```python
from build123d import *

# Parameters (mm, degrees)
SKETCH1_W           = 100
SKETCH1_H           = 100
SKETCH1_R           = 2.75
BOSS_EXTRUDE1_DEPTH = 4.3
SKETCH2_R           = 1.75
BOSS_EXTRUDE2_DEPTH = 4.3
FILLET1_R           = 10


with BuildPart() as part:
    # Sketch1 → Boss-Extrude1 (new body)
    with BuildSketch(Plane(origin=(0, 0, 0), x_dir=(1, 0, 0), z_dir=(0, 1, 0))):
        with Locations((50, 50)):
            Rectangle(SKETCH1_W, SKETCH1_H)
        with Locations((20, 80)):
            Circle(SKETCH1_R, mode=Mode.SUBTRACT)
        with Locations((80, 80)):
            Circle(SKETCH1_R, mode=Mode.SUBTRACT)
        with Locations((80, 20)):
            Circle(SKETCH1_R, mode=Mode.SUBTRACT)
        with Locations((20, 20)):
            Circle(SKETCH1_R, mode=Mode.SUBTRACT)
    extrude(amount=BOSS_EXTRUDE1_DEPTH)

    # Sketch2 → Boss-Extrude2 (add)
    with BuildSketch(Plane(origin=(0, 4.3, 0), x_dir=(1, 0, 0), z_dir=(0, 1, 0))):
        with BuildLine():
            Line((0, 80.554563517), (-44.722718241, 125.277281759))
            ThreePointArc((-44.722718241, 125.277281759), (-44.722718241, 144.722718241), (-25.277281759, 144.722718241))
            Line((-25.277281759, 144.722718241), (19.445436483, 100))
            Line((19.445436483, 100), (0, 100))
            Line((0, 100), (0, 80.554563517))
        make_face()
        with Locations((-35, 135)):
            Circle(SKETCH2_R, mode=Mode.SUBTRACT)
        with BuildLine():
            Line((100, 100), (100, 80.554563517))
            Line((100, 80.554563517), (144.722718241, 125.277281759))
            ThreePointArc((144.722718241, 125.277281759), (144.722718241, 144.722718241), (125.277281759, 144.722718241))
            Line((125.277281759, 144.722718241), (80.554563517, 100))
            Line((80.554563517, 100), (100, 100))
        make_face()
        with Locations((135, 135)):
            Circle(SKETCH2_R, mode=Mode.SUBTRACT)
        with BuildLine():
            Line((100, 0), (80.554563517, 0))
            Line((80.554563517, 0), (125.277281759, -44.722718241))
            ThreePointArc((125.277281759, -44.722718241), (144.722718241, -44.722718241), (144.722718241, -25.277281759))
            Line((144.722718241, -25.277281759), (100, 19.445436483))
            Line((100, 19.445436483), (100, 0))
        make_face()
        with Locations((135, -35)):
            Circle(SKETCH2_R, mode=Mode.SUBTRACT)
        with BuildLine():
            Line((0, 0), (0, 19.445436483))
            Line((0, 19.445436483), (-44.722718241, -25.277281759))
            ThreePointArc((-44.722718241, -25.277281759), (-44.722718241, -44.722718241), (-25.277281759, -44.722718241))
            Line((-25.277281759, -44.722718241), (19.445436483, 0))
            Line((19.445436483, 0), (0, 0))
        make_face()
        with Locations((-35, -35)):
            Circle(SKETCH2_R, mode=Mode.SUBTRACT)
    extrude(amount=-BOSS_EXTRUDE2_DEPTH)

    # Fillet1
    fillet1_edges = [part.edges().sort_by_distance(p)[0] for p in [
        (0, 2.15, -80.554563517),
        (19.445436483, 2.15, -100),
        (80.554563517, 2.15, -100),
        (100, 2.15, -80.554563517),
        (100, 2.15, -19.445436483),
        (80.554563517, 2.15, 0),
        (19.445436483, 2.15, 0),
        (0, 2.15, -19.445436483),
    ]]
    fillet(fillet1_edges, radius=FILLET1_R)


solid = part.part
```
The model under review builds one solid part; all positions refer to its coordinate system, in mm. A direction names the side the tool comes from. Round coordinates to 2 decimals unless told otherwise and drop trailing zeros. Order: outer loops, then holes, each group sorted by start corner. A loop starts at its lowest first (then second) coordinate and runs counter-clockwise, first axis right, second up. Notation, with made-up numbers: (74, -20) - (132, -20) arc R27 cw to (132, 16) - close; hole circle Ø4 at (-21.5, 36.5). An arc over 180 degrees is marked (long way). Answer in a Markdown table with one row per item.
(1) Take a section at B-B on x = 107. Write out the cut boundary in (y, z).
Result set:
| item | result |
|---|---|
| outline | (0, -126.45) - (4.3, -126.45) - (4.3, -87.55) - (0, -87.55) - close; (0, -12.45) - (4.3, -12.45) - (4.3, 26.45) - (0, 26.45) - close |
(2) Machinability: for faces 5 (the face through (80.19, 2.12, -100.74)), 6 (the face through (17.253, 2.12, -80.121)), 7 (the face through (100, 2, -50)), 8 (the face through (51, 4.3, -51)), 9 (the face through (19.81, 2.12, 0.74)), which of the approach directions +Z, -Z, +X, -X, +Y, -Y give a long, thin tool a straight path to every point of the face, cutting with its end or side? Answer none if there is none.
Result set:
| item | result |
|---|---|
| face 5 | -Z, +Y, -Y |
| face 6 | +Y, -Y |
| face 7 | +X, +Y, -Y |
| face 8 | +Z, -Z, +X, -X, +Y |
| face 9 | +Z, +Y, -Y |
(3) Take a section at D-D on x = 20. Write out the cut boundary in (y, z).
Result set:
| item | result |
|---|---|
| outline | (0, -100.67) - (4.3, -100.67) - (4.3, -82.75) - (0, -82.75) - close; (0, -77.25) - (4.3, -77.25) - (4.3, -22.75) - (0, -22.75) - close; (0, -17.25) - (4.3, -17.25) - (4.3, 0.67) - (0, 0.67) - close |
(4) Take a section at C-C on z = 12. Write out the cut boundary in (x, y), plus the area to 3 significant figures.
Result set:
| item | result |
|---|---|
| outline | (-31.45, 0) - (7.45, 0) - (7.45, 4.3) - (-31.45, 4.3) - close; (92.55, 0) - (131.45, 0) - (131.45, 4.3) - (92.55, 4.3) - close |
| area | 334 mm2 |
(5) Mouldability with a two-part tool opening along X and no side actions: class faces 1 (the face through (100.74, 2.12, -80.19)), 2 (the face through (50, 2, 0)), 3 (the face through (-0.74, 2.12, -19.81)), 4 (the face through (144.51, 2.18, 44.93)) as released by +X, released by -X, zero draft, split by the parting line, or undercut.
Result set:
| item | result |
|---|---|
| face 1 | released by +X |
| face 2 | undercut |
| face 3 | released by -X |
| face 4 | undercut |
(6) Take a section at A-A on y = 2.15. Count the separate pieces of the cut face and the enclosed holes in it, plus the area to 3 significant figures.
Result set:
| item | result |
|---|---|
| separate pieces | 1 |
| enclosed holes | 8 |
| area | 17,300 mm2 |
(7) For line 1 (Z direction, x = -35, y = 3.3); line 2 (X direction, y = 3.1, z = 35); line 3 (X direction, y = 1.25, z = -20), list the stretches that pass through material, from the lowest coordinate up. Write a range as from..to.
Result set:
| item | result |
|---|---|
| line 1 | z = -148.75..-136.75, -133.25..-115.55, 15.55..33.25, 36.75..48.75 |
| line 2 | x = -48.75..-36.75, -33.25..-15.55, 115.55..133.25, 136.75..148.75 |
| line 3 | x = -0.67..17.25, 22.75..77.25, 82.75..100.67 |
(8) Clearance check with flat-ended pins moving along their axes: P1, Ø1.5, axis at x = 80.5, y = 2.5, coming from the +Z side; P2, Ø2, axis at x = 82, y = 1, coming from the +Z side; P3, Ø2, axis at x = 50.5, y = 2, coming from the +Z side. State where each tip first meets the part, or that it passes through.
Result set:
| item | result |
|---|---|
| P1 | stops at z = 1.25 |
| P2 | stops at z = 2.48 |
| P3 | stops at z = 0 |
